Input: part model. Units: mm. Frame: model coordinates. A direction names the side the tool comes from. Coordinates: 2 decimals unless noted, no trailing zeros. Loops run counter-clockwise (first coordinate to the right, second up) from the corner with the lowest first, then second, coordinate; pieces in that order, holes last. Notation, with made-up numbers: (8, -25) -> (16, -25) arc R14 ccw to (16, -1) -> close; hole circle Ø6 at (-27.5, -32.5). An arc over 180 degrees is marked (long way). Answer as a JSON object with one key per item and string values.
from build123d import *

# Parameters (mm, degrees)
ESQUISSE1_W             = 49
ESQUISSE1_H             = 80
BOSS_EXTRU_1_DEPTH      = 50
ESQUISSE2_W             = 73.004277741
ESQUISSE2_H             = 90.842499223
ENL_V_MAT_EXTRU_1_DEPTH = 101
D_GAGEMENT_M61_D        = 6.6
D_GAGEMENT_M241_D       = 26


with BuildPart() as part:
    # Esquisse1 → Boss.-Extru.1 (new body)
    with BuildSketch(Plane.XY):
        Rectangle(ESQUISSE1_W, ESQUISSE1_H)
    extrude(amount=BOSS_EXTRU_1_DEPTH)

    # Esquisse2 → Enlèv. mat.-Extru.1 (cut)
    with BuildSketch(Plane(origin=(24.5, 0, 0), x_dir=(0, 0, -1), z_dir=(1, 0, 0))):
        with Locations((-41.502138871, 10.421249612)):
            Rectangle(ESQUISSE2_W, ESQUISSE2_H)
    extrude(amount=-ENL_V_MAT_EXTRU_1_DEPTH, mode=Mode.SUBTRACT)

    # Dégagement M61 (through all)
    with Locations(Plane(origin=(0, -40, 0), x_dir=(-1, 0, 0), z_dir=(0, -1, 0))):
        with Locations((-12.051490403, -21.293816609), (12.769236225, -21.293816609)):
            Hole(D_GAGEMENT_M61_D / 2)

    # Dégagement M241 (through all)
    with Locations(Plane.XY.offset(5)):
        with Locations((-0.37, 4.133244148)):
            Hole(D_GAGEMENT_M241_D / 2)


solid = part.part
1. Line query: line 1 along Y through (x, z) = (14, 11); line 2 along Z through (x, y) = (-22, -6); line 3 along Y through (x, z) = (-0.37, 2.9). Output: solid intervals per line, ascending.
Reply:
{"line 1": "y = -40 to -35", "line 2": "z = 0 to 5", "line 3": "y = -40 to -8.87, 17.13 to 40"}
2. Section query C-C (y = -16.5). Return loops of the section in (x, z), plus the area to 3 significant figures.
Reply:
{"outline": "(-24.5, 0) -> (24.5, 0) -> (24.5, 5) -> (-24.5, 5) -> close", "area": "245 mm2"}
3. Section query B-B (x = 11). Return loops of the section in (y, z), plus the area to 3 significant figures.
Reply:
{"outline": "(-40, 0) -> (-2.17, 0) -> (-2.17, 5) -> (-35, 5) -> (-35, 18.17) -> (-40, 18.17) -> close; (-40, 24.42) -> (-35, 24.42) -> (-35, 50) -> (-40, 50) -> close; (10.44, 0) -> (40, 0) -> (40, 5) -> (10.44, 5) -> close", "area": "531 mm2"}
4. Section query D-D (z = 10). Return loops of the section in (x, y), plus the area to 3 significant figures.
Reply:
{"outline": "(-24.5, -40) -> (24.5, -40) -> (24.5, -35) -> (-24.5, -35) -> close", "area": "245 mm2"}
5. Mould query, pull axis X, two halves, no side actions, for faces 3 (the face through (0, -35, 28)), 4 (the face through (-12.77, 8.04, 2.47)), 5 (the face through (-13.485, -37.465, 24.515)), 6 (the face through (-24.5, -18, 4.5)). Classes: pulls with the +X half, pulls with the -X half, needs draft (parallel to the pull), parting line crosses it, or undercut.
Reply:
{"face 3": "needs draft", "face 4": "undercut", "face 5": "undercut", "face 6": "pulls with the -X half"}
6. Pin query (flat end, axial travel): P1, Ø5, axis at x = -11, y = 11.5, coming from the +Z side; P2, Ø4, axis at x = -10, z = 27, coming from the +Y side. Return the tip coordinate at first contact, or that it passes through.
Reply:
{"P1": "stops at z = 5", "P2": "stops at y = -35"}
7. Access query for faces 1 (the face through (0, -40, 25)), 2 (the face through (11, -6, 5)). Directions: +Z, -Z, +X, -X, +Y, -Y. A direction counts if a zero-diameter tool reaches every point of the face in a straight line with its end or side. Return the directions, or none.
Reply:
{"face 1": "+Z, -Z, +X, -X, -Y", "face 2": "+Z, +X, -X, +Y"}
8. Section query A-A (x = -0.37). Return loops of the section in (y, z), plus the area to 3 significant figures.
Reply:
{"outline": "(-40, 0) -> (-8.87, 0) -> (-8.87, 5) -> (-35, 5) -> (-35, 50) -> (-40, 50) -> close; (17.13, 0) -> (40, 0) -> (40, 5) -> (17.13, 5) -> close", "area": "495 mm2"}
